```python
from build123d import *

# Parameters (mm, degrees)
SKETCH1_W                      = 23
SKETCH1_H                      = 8
BOSS_EXTRUDE1_DEPTH            = 8
SKETCH2_R                      = 5
CUT_EXTRUDE1_DEPTH             = 15.568802284
CBORE_FOR_M3_SHCS1_D           = 3.4
CBORE_FOR_M3_SHCS1_CBORE_D     = 5.8
CBORE_FOR_M3_SHCS1_CBORE_DEPTH = 3
SKETCH8_R                      = 3.25
CUT_EXTRUDE2_DEPTH             = 15.568802284
FILLET1_R                      = 1.5


with BuildPart() as part:
    # Sketch1 → Boss-Extrude1 (new body)
    with BuildSketch(Plane.XY):
        Rectangle(SKETCH1_W, SKETCH1_H)
    extrude(amount=BOSS_EXTRUDE1_DEPTH)

    # Sketch2 → Cut-Extrude1 (cut, through all)
    with BuildSketch(Plane(origin=(0, 0, 0), x_dir=(1, 0, 0), z_dir=(0, 1, 0))):
        Circle(SKETCH2_R)
    extrude(amount=-CUT_EXTRUDE1_DEPTH, mode=Mode.SUBTRACT)

    # CBORE for M3 SHCS1 (through all)
    with Locations(Plane.XY.offset(8)):
        with Locations((-8, 0), (8, 0)):
            CounterBoreHole(CBORE_FOR_M3_SHCS1_D / 2, CBORE_FOR_M3_SHCS1_CBORE_D / 2, CBORE_FOR_M3_SHCS1_CBORE_DEPTH)

    # Sketch8 → Cut-Extrude2 (cut, through all)
    with BuildSketch(Plane(origin=(0, 0, 0), x_dir=(1, 0, 0), z_dir=(0, 1, 0))):
        Circle(SKETCH8_R)
    extrude(amount=CUT_EXTRUDE2_DEPTH, mode=Mode.SUBTRACT)

    # Fillet1
    # the kernel refuses this fillet: 1.5 mm, written as the material it takes off along each edge
    with BuildSketch(Plane(origin=(-11.5, -7.75, 8), x_dir=(1, 0, 0), z_dir=(0, 1, 0))) as fillet1_piece_1:
        with BuildLine():
            CenterArc((FILLET1_R, FILLET1_R), FILLET1_R, 180, 90)
            Line((0, FILLET1_R), (0, 0))
            Line((0, 0), (FILLET1_R, 0))
        make_face()
    extrude(amount=15.5, mode=Mode.SUBTRACT)
    with BuildSketch(Plane(origin=(11.5, 7.75, 8), x_dir=(0, 0, -1), z_dir=(0, -1, 0))) as fillet1_piece_2:
        with BuildLine():
            CenterArc((FILLET1_R, -FILLET1_R), FILLET1_R, 90, 90)
            Line((0, -FILLET1_R), (0, 0))
            Line((0, 0), (FILLET1_R, 0))
        make_face()
    extrude(amount=15.5, mode=Mode.SUBTRACT)


solid = part.part
```
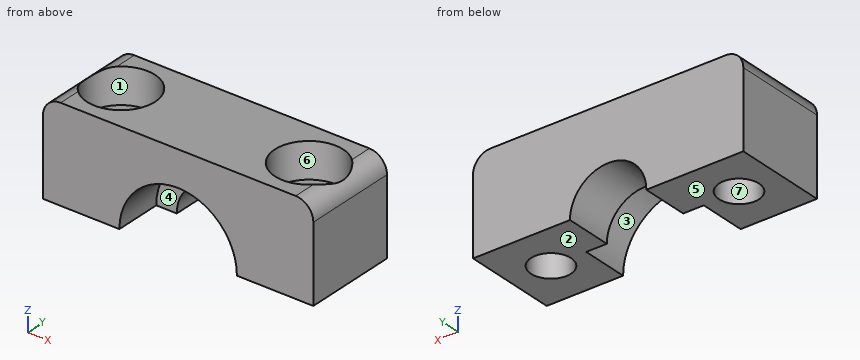
The model under review builds one solid part; all positions refer to its coordinate system, in mm. Face numbers are marked on the shaded views. A direction names the side the tool comes from. Coordinates: 2 decimals unless noted, no trailing zeros. Order: outer loops, then holes, each group sorted by start corner. A loop starts at its lowest first (then second) coordinate and runs counter-clockwise, first axis right, second up. Notation, with made-up numbers: (-3, 21) -> (49, 21) arc R11 ccw to (49, 35) -> close; hole circle Ø6 at (20.5, 12.25). An arc over 180 degrees is marked (long way). Answer in a Markdown table with one row per item. Add a question column.
Item 1: Mouldability with a two-part tool opening along Y and no side actions: class the marked faces 4, 5, 6 and 7 as +Y half, -Y half, draft (parallel to the pull), parting line (faces both ways), or undercut.
Item 2: To check wall thickness, follow probe 1 along Y at (x, z) = (-8, 1.6); probe 2 along X at (y, z) = (-0.5, 6.25); probe 3 along Y at (x, z) = (-8, 6.25). State the ranges of each line that lie inside material, in increasing order.
Item 3: Clearance check with flat-ended pins moving along their axes: pin 1 (1.5 mm diameter, centred on x = 2.5, z = 1.5, fed in from -Y); pin 2 (2.5 mm diameter, centred on x = 8, y = 0, fed in from +Z). State where each tip first meets the part, or that it passes through.
Item 4: We need section D-D on z = 6. Write out the cut boundary in (x, y), plus the area to 3 significant figures.
Item 5: We need section C-C on y = -0.25. Write out the cut boundary in (x, z), plus the area to 3 significant figures.
Item 6: Machinability: for the marked faces 1, 2 and 3, which of the approach directions +Z, -Z, +X, -X, +Y, -Y give a long, thin tool a straight path to every point of the face, cutting with its end or side? Answer none if there is none.
Item 7: We need section A-A on z = 2.75. Write out the cut boundary in (x, y), plus the area to 3 significant figures.
Item 8: We need section B-B on x = -8. Write out the cut boundary in (y, z), plus the area to 3 significant figures.
Final values:
| question | item | result |
|---|---|---|
| 1 | face 4 | -Y half |
| 1 | face 5 | draft |
| 1 | face 6 | undercut |
| 1 | face 7 | undercut |
| 2 | probe 1 | y = -4 to -1.7, 1.7 to 4 |
| 2 | probe 2 | x = -11.5 to -10.86, -5.14 to 5.14, 10.86 to 11.5 |
| 2 | probe 3 | y = -4 to -2.9, 2.9 to 4 |
| 3 | pin 1 | stops at y = 0 |
| 3 | pin 2 | passes through |
| 4 | outline | (-11.5, -4) -> (11.5, -4) -> (11.5, 4) -> (-11.5, 4) -> close; hole circle Ø5.8 at (-8, 0); hole circle Ø5.8 at (8, 0) |
| 4 | area | 131 mm2 |
| 5 | outline | (-11.5, 0) -> (-9.68, 0) -> (-9.68, 5) -> (-10.89, 5) -> (-10.89, 7.71) arc R1.5 ccw to (-11.5, 6.5) -> close; (-6.32, 0) -> (-5, 0) arc R5 cw to (5, 0) -> (6.32, 0) -> (6.32, 5) -> (5.11, 5) -> (5.11, 8) -> (-5.11, 8) -> (-5.11, 5) -> (-6.32, 5) -> close; (9.68, 0) -> (11.5, 0) -> (11.5, 6.5) arc R1.5 ccw to (10.89, 7.71) -> (10.89, 5) -> (9.68, 5) -> close |
| 5 | area | 75.6 mm2 |
| 6 | face 1 | +Z |
| 6 | face 2 | -Z, +X, -X, +Y, -Y |
| 6 | face 3 | -Z, -Y |
| 7 | outline | (-11.5, -4) -> (-4.18, -4) -> (-4.18, 0) -> (-1.73, 0) -> (-1.73, 4) -> (-11.5, 4) -> close; (1.73, 0) -> (4.18, 0) -> (4.18, -4) -> (11.5, -4) -> (11.5, 4) -> (1.73, 4) -> close; hole circle Ø3.4 at (-8, 0); hole circle Ø3.4 at (8, 0) |
| 7 | area | 119 mm2 |
| 8 | outline | (-4, 0) -> (-1.7, 0) -> (-1.7, 5) -> (-2.9, 5) -> (-2.9, 8) -> (-4, 8) -> close; (1.7, 0) -> (4, 0) -> (4, 8) -> (2.9, 8) -> (2.9, 5) -> (1.7, 5) -> close |
| 8 | area | 29.6 mm2 |
